```python
from build123d import *

# Parameters (mm, degrees)
SKETCH1_W             = 40
SKETCH1_H             = 40
BOSS_EXTRUDE1_DEPTH   = 48
M4X0_7_TAPPED_HOLE1_D = 3.3
SKETCH10_W            = 40
SKETCH10_H            = 20
CUT_EXTRUDE4_DEPTH    = 49
SKETCH11_W            = 11.25
SKETCH11_H            = 7.2
CUT_EXTRUDE5_REACH    = 50
SKETCH12_R            = 10
M4X0_7_TAPPED_HOLE2_D = 3.3
SKETCH15_W            = 40
SKETCH15_H            = 7.5
CUT_EXTRUDE6_DEPTH    = 36
SKETCH16_W            = 5
SKETCH16_H            = 5
CUT_EXTRUDE7_DEPTH    = 13


with BuildPart() as part:
    # Sketch1 → Boss-Extrude1 (new body)
    with BuildSketch(Plane(origin=(0, 0, 0), x_dir=(1, 0, 0), z_dir=(0, 1, 0))):
        Rectangle(SKETCH1_W, SKETCH1_H)
    extrude(amount=-BOSS_EXTRUDE1_DEPTH)

    # M4x0.7 Tapped Hole1 (through all)
    with Locations(Plane(origin=(0, 0, 0), x_dir=(1, 0, 0), z_dir=(0, 1, 0))):
        with Locations((-15.5, 15), (15.5, 15), (15.5, -15), (-15.5, -15)):
            Hole(M4X0_7_TAPPED_HOLE1_D / 2)

    # Sketch10 → Cut-Extrude4 (cut, through all)
    with BuildSketch(Plane(origin=(0, 0, 0), x_dir=(1, 0, 0), z_dir=(0, 1, 0))):
        with Locations((0, -10)):
            Rectangle(SKETCH10_W, SKETCH10_H)
    extrude(amount=-CUT_EXTRUDE4_DEPTH, mode=Mode.SUBTRACT)

    # Sketch11 → Cut-Revolve2 (revolve, cut)
    with BuildSketch(Plane.XY):
        with Locations((5.625, -43.6)):
            Rectangle(SKETCH11_W, SKETCH11_H)
    revolve(axis=Axis((0, 0, 0), (0, -1, 0)), mode=Mode.SUBTRACT)

    # Sketch12 → Cut-Extrude5 (cut, up to next)
    with BuildSketch(Plane.XZ.offset(48), mode=Mode.PRIVATE) as cut_extrude5_sk1:
        Circle(SKETCH12_R)
    cut_extrude5_tool1 = extrude(cut_extrude5_sk1.sketch, amount=-CUT_EXTRUDE5_REACH, mode=Mode.PRIVATE) & part.part
    add(cut_extrude5_tool1.solids().sort_by_distance((0, -48, 0))[0], mode=Mode.SUBTRACT)

    # M4x0.7 Tapped Hole2 (through all)
    with Locations(Plane(origin=(0, 0, -20), x_dir=(-1, 0, 0), z_dir=(0, 0, -1))):
        with Locations((15, -43.628125), (-15, -43.628125), (0, -36.484375), (0, -18.2421875)):
            Hole(M4X0_7_TAPPED_HOLE2_D / 2)

    # Sketch15 → Cut-Extrude6 (cut)
    with BuildSketch(Plane.XZ.offset(48)):
        with Locations((0, -16.25)):
            Rectangle(SKETCH15_W, SKETCH15_H)
    extrude(amount=-CUT_EXTRUDE6_DEPTH, mode=Mode.SUBTRACT)

    # Sketch16 → Cut-Extrude7 (cut, through all)
    with BuildSketch(Plane.XZ.offset(12)):
        with Locations((0, -17.5)):
            Rectangle(SKETCH16_W, SKETCH16_H)
    extrude(amount=-CUT_EXTRUDE7_DEPTH, mode=Mode.SUBTRACT)


solid = part.part
```
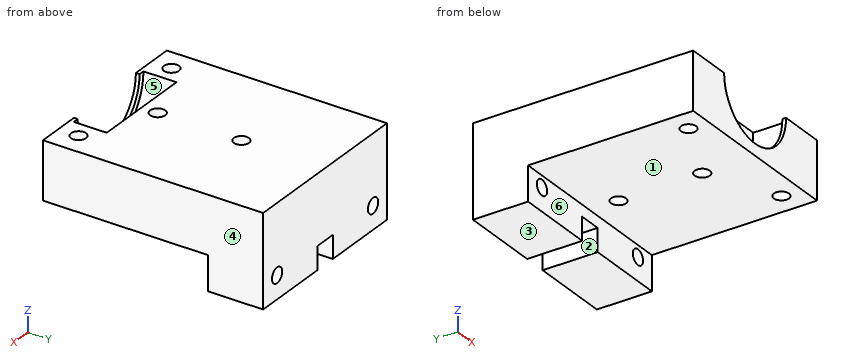
Check sheet for the modelled part. Datum: model origin and axes. Units: mm. Face numbers are marked on the shaded views. A direction names the side the tool comes from. Coordinates: 2 decimals unless noted, no trailing zeros. Write each loop counter-clockwise with the first axis right and the second up, starting at its lowest first coordinate (ties: lowest second). Pieces come first, ordered by that corner, then holes. Notation, with made-up numbers: (-19.5, 58.25) -> (1.5, 58.25) arc R20 ccw to (1.5, 90.25) -> close; hole circle Ø6 at (-9.5, 15.5). An arc over 180 degrees is marked (long way). Use a Markdown table: item, result.
1. Sectioned sample at C-C (x = -15). Enter the section's corners in (y, z).
Reported:
| item | result |
|---|---|
| outline | (-48, -12.5) -> (-45.28, -12.5) -> (-45.28, 0) -> (-48, 0) -> close; (-41.98, -12.5) -> (-12, -12.5) -> (-12, -13.43) -> (0, -13.43) -> (0, 0) -> (-41.98, 0) -> close; (-12, -20) -> (0, -20) -> (0, -16.57) -> (-12, -16.57) -> close |
2. Tool access check on the marked faces 1, 2 and 3. Record the directions out of +Z, -Z, +X, -X, +Y, -Y that give a thin tool (end or side, any length) a straight path to the whole face; none if there is none.
Reported:
| item | result |
|---|---|
| face 1 | -Z, +X, -X, -Y |
| face 2 | -Z, +Y, -Y |
| face 3 | -Z, +X, -X, +Y, -Y |
3. Sectioned sample at B-B (y = -4). Enter the section's corners in (x, z), plus the area to 3 significant figures.
Reported:
| item | result |
|---|---|
| outline | (-20, -20) -> (-2.5, -20) -> (-2.5, -15) -> (2.5, -15) -> (2.5, -20) -> (20, -20) -> (20, 0) -> (-20, 0) -> close; hole circle Ø3.3 at (-15.5, -15); hole circle Ø3.3 at (15.5, -15) |
| area | 758 mm2 |
4. Sectioned sample at D-D (z = -8.25). Enter the section's corners in (x, y), plus the area to 3 significant figures.
Reported:
| item | result |
|---|---|
| outline | (-20, -48) -> (-5.65, -48) -> (-5.65, -47.2) -> (-7.65, -47.2) -> (-7.65, -40) -> (7.65, -40) -> (7.65, -47.2) -> (5.65, -47.2) -> (5.65, -48) -> (20, -48) -> (20, 0) -> (-20, 0) -> close; hole circle Ø3.3 at (-15, -43.63); hole circle Ø3.3 at (0, -36.48); hole circle Ø3.3 at (0, -18.24); hole circle Ø3.3 at (15, -43.63) |
| area | 1,770 mm2 |
5. Release check for a two-part mould opening along Y. For the marked faces 4, 5 and 6 record: pulls with the +Y half, pulls with the -Y half, needs draft (parallel to the pull), parting line crosses it, or undercut.
Reported:
| item | result |
|---|---|
| face 4 | needs draft |
| face 5 | undercut |
| face 6 | pulls with the -Y half |
6. Scan lines: line 1 along Y through (x, z) = (0, -9.25); line 2 along Z through (x, y) = (15.5, -4.75); line 3 along X through (y, z) = (-42.5, -1.5). Record each from-to range of solid material in increasing order.
Reported:
| item | result |
|---|---|
| line 1 | y = -40 to -38.13, -34.83 to -19.89, -16.59 to 0 |
| line 2 | z = -20 to -16.65, -13.35 to 0 |
| line 3 | x = -20 to -16.2, -13.8 to -11.15, 11.15 to 13.8, 16.2 to 20 |
7. Go/stop test with flat-tipped pins: pin 1 Ø5.5 at (x, y) = (-15, -43.63) entering from -Z; pin 2 Ø2 at (y, z) = (-18, -14) entering from +X; pin 3 Ø3.5 at (x, z) = (-5.5, -3.5) entering from -Y; pin 4 Ø2.5 at (x, y) = (1, -7) entering from -Z. Record where each tip stops, or that it passes through.
Reported:
| item | result |
|---|---|
| pin 1 | stops at z = -12.5 |
| pin 2 | passes through |
| pin 3 | stops at y = -40 |
| pin 4 | stops at z = -15 |
8. Sectioned sample at A-A (z = -18.5). Enter the section's corners in (x, y), plus the area to 3 significant figures.
Reported:
| item | result |
|---|---|
| outline | (-20, -12) -> (-2.5, -12) -> (-2.5, 0) -> (-20, 0) -> close; (2.5, -12) -> (20, -12) -> (20, 0) -> (2.5, 0) -> close |
| area | 420 mm2 |
